Check sheet for the modelled part. Datum: model origin and axes. Units: mm. Face numbers are marked on the shaded views. Coordinates: 2 decimals unless noted, no trailing zeros. Loops run counter-clockwise (first coordinate to the right, second up) from the corner with the lowest first, then second, coordinate; pieces in that order, holes last. Notation, with made-up numbers: (-16.75, -14.5) -> (14.25, -14.5) arc R34 cw to (14.25, 24.5) -> close; hole circle Ø10 at (42.5, 86). An arc over 180 degrees is marked (long way). Use one line per item in the form item = value.
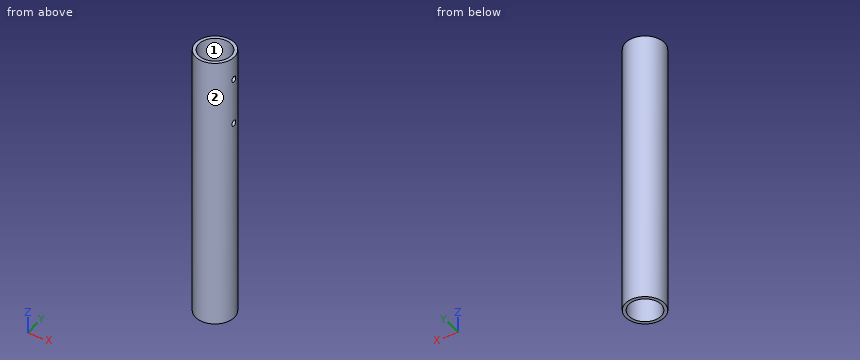
Autodesk Inventor part; units mm, degrees
ref_plane "Work Plane1" through (0, 0, 0) normal (1, 0, 0) x (0, 0, 1)
ref_plane "XZ Plane" through (0, 0, 0) normal (0, 1, 0) x (-1, 0, 0)
ref_plane "XY Plane" through (0, 0, 0) normal (0, 0, 1) x (1, 0, 0)
sketch "Sketch1" plane through (0, 0, 0) normal (0, 0, 1) x (1, 0, 0)
  circle A0 centre (0, 0) radius 21.0312
  circle A1 centre (0, 0) radius 17.4625
  dimension "d0" = 42.0624
  dimension "d1" = 34.925
extrude "Extrusion1" add sketch "Sketch1" along normal blind 301.625
ref_plane "Work Plane1" through (0, 0, 0) normal (1, 0, 0) x (0, 0, 1)
sketch "Sketch2" plane through (0, 0, 0) normal (1, 0, 0) x (0, 0, 1)
  line L0 (0, -21.0312) -> (301.625, -21.0312)
  line L1 (0, 21.0312) -> (301.625, 21.0312)
  line L2 (301.625, 17.4625) -> (301.625, -17.4625)
  line L3 (301.625, 21.0312) -> (301.625, -21.0312)
  line L4 (-60.325, 0) -> (361.95, 0)
  circle A0 centre (276.225, 0) radius 3.175
  dimension "d5" = 25.4
  dimension "d6" = 6.35
extrude "Extrusion2" cut sketch "Sketch2" along normal blind 50.8
pattern_linear "Rectangular Pattern1" count 2 spacing 50.8 along (0, 0, -1) of "Extrusion2"
properties part number "FE-00006-02"
(1) Mould release check, pull along X, two halves, no side actions. Record for the marked faces 1 and 2: +X half, -X half, draft (parallel to the pull), parting line (faces both ways), or undercut.
Established:
face_1 = undercut
face_2 = parting line
(2) Section check C-C, the plane y = 13. Record the boundary of the cut face in (x, z) (3 decimals), plus the area to 3 significant figures.
Established:
outline = (-16.532, 0) -> (-11.659, 0) -> (-11.659, 301.625) -> (-16.532, 301.625) -> close; (11.659, 0) -> (16.532, 0) -> (16.532, 301.625) -> (11.659, 301.625) -> close
area = 2,940 mm²
(3) Section check A-A, the plane y = 0. Give the number of separate pieces and of enclosed holes in the cut face, plus the area to 3 significant figures.
Established:
separate_pieces = 4
enclosed_holes = 0
area = 2,110 mm²
(4) Scan lines: line 1 along Z through (x, y) = (18.3, 0) (3 decimals); line 2 along Y through (x, z) = (0, 141); line 3 along Y through (x, z) = (-15.5, 73.5). Record each from-to range of solid material in increasing order.
Established:
line_1 = 0 to 222.25, 228.6 to 273.05, 279.4 to 301.625
line_2 = -21.03 to -17.46, 17.46 to 21.03
line_3 = -14.21 to -8.04, 8.04 to 14.21
(5) Go/stop test with flat-tipped pins: P1, Ø1.5, axis at y = -12.5, z = 62, coming from the +X side; P2, Ø2, axis at y = -12.5, z = 164, coming from the +X side; P3, Ø8, axis at x = -1.5, z = 202, coming from the +Y side. Record where each tip stops, or that it passes through.
Established:
P1 = 17.44
P2 = 17.61
P3 = 21.03
(6) Section check B-B, the plane x = 0. Record the boundary of the cut face in (y, z) (1 decimal).
Established:
outline = (-21, 0) -> (-17.5, 0) -> (-17.5, 301.6) -> (-21, 301.6) -> close; (17.5, 0) -> (21, 0) -> (21, 301.6) -> (17.5, 301.6) -> close
(7) Section check D-D, the plane z = 71.5. Record the boundary of the cut face in (x, y) (1 decimal), plus the area to 3 significant figures.
Established:
outline = circle Ø42.1 at (0, 0); hole circle Ø34.9 at (0, 0)
area = 432 mm²
